Here's how the part is built. I have some questions about the finished solid (model axes, mm). Face numbers are marked on the shaded views. A direction names the side the tool comes from. Round coordinates to 2 decimals unless told otherwise and drop trailing zeros. Loops run counter-clockwise (first coordinate to the right, second up) from the corner with the lowest first, then second, coordinate; pieces in that order, holes last. Notation, with made-up numbers: M -36,-23 L 11,-23 A26 cw 11,-4 Z; hole C 19,39.25 d3. An arc over 180 degrees is marked long. Answer as a JSON object with one key per item and string values.
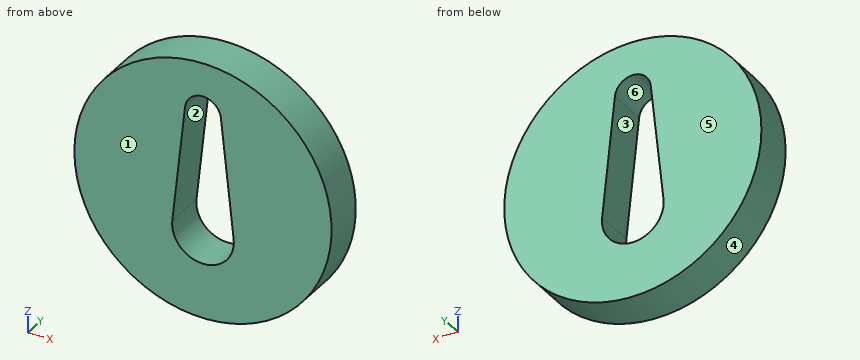
Autodesk Inventor part; units mm, degrees
ref_plane "YZ Plane" through (0, 0, 0) normal (1, 0, 0) x (0, 1, 0)
ref_plane "XZ Plane" through (0, 0, 0) normal (0, 1, 0) x (-1, 0, 0)
ref_plane "XY Plane" through (0, 0, 0) normal (0, 0, 1) x (1, 0, 0)
sketch "Sketch1" plane through (0, 0, 0) normal (0, 1, 0) x (-1, 0, 0)
  circle A0 centre (0, 0) radius 20 construction
  circle A1 centre (0, 5) radius 15
  circle A2 centre (0, 0) radius 3.5
  circle A3 centre (0, 14) radius 2
  line L0 (-1.9885, 14.2143) -> (-3.4799, 0.375)
  line L1 (1.9885, 14.2143) -> (3.4799, 0.375)
  dimension "d0" = 40
  dimension "d1" = 30
  dimension "d2" = 7
  dimension "d3" = 4
  dimension "d4" = 19.5
extrude "Extrusion1" add sketch "Sketch1" along normal blind 4.8
sketch "Sketch2" plane through (0, 4.8, 5) normal (0, 1, 0) x (1, 0, 0)
  arc A0 (-1.9885, -9.2143) -> (1.9885, -9.2143) centre (0, -9) ccw
  line L0 (1.9885, -9.2143) -> (3.4799, 4.625)
  arc A1 (3.4799, 4.625) -> (-3.4799, 4.625) centre (0, 5) ccw
  line L1 (-3.4799, 4.625) -> (-1.9885, -9.2143)
  circle A2 centre (0, 0) radius 15
  arc A3 (-2.0879, -9.225) -> (2.0879, -9.225) centre (0, -9) ccw
  line L2 (2.0879, -9.225) -> (3.5793, 4.6143)
  arc A4 (3.5793, 4.6143) -> (-3.5793, 4.6143) centre (0, 5) ccw
  line L3 (-3.5793, 4.6143) -> (-2.0879, -9.225)
  dimension "d7" = 0.1
extrude "Extrusion2" cut sketch "Sketch2" against normal through all contours L3 A4 L2 A3
properties part number "Ventil Scheibe_3DPrint"
Item 1: I want a section at B-B on x = 0. List the corners of the cut face in (y, z) for me, plus the area to 3 significant figures.
Solution:
{"outline": "M 0,-10 L 4.8,-10 L 4.8,-3.6 L 0,-3.6 Z; M 0,16.1 L 4.8,16.1 L 4.8,20 L 0,20 Z", "area": "49.4 mm2"}
Item 2: We'd pull the mould along Z, two halves only. Please class the marked faces 1, 2, 3 and 4: +Z half, -Z half, draft (parallel to the pull), parting line (faces both ways), or undercut.
Solution:
{"face 1": "draft", "face 2": "undercut", "face 3": "undercut", "face 4": "parting line"}
Item 3: If I drill on L1, parallel to X at y = 1.5, z = 13.5; L2, parallel to X at y = 3.25, z = 0; L3, parallel to Z at x = 10, y = 1.3, over which ranges is the centre line in solid material (lowest first)? Write a range as from..to.
Solution:
{"L1": "x = -12.36..-2.17, 2.17..12.36", "L2": "x = -14.14..-3.6, 3.6..14.14", "L3": "z = -6.18..16.18"}
Item 4: For P1, Ø2, axis at x = 6, y = 3.5, coming from the -Z side, with a flat end and sliding along its axis, tell me the tip position at first contact or that it passes through.
Solution:
{"P1": "stops at z = -9.14"}
Item 5: I want a section at D-D on z = -7. List the corners of the cut face in (x, y) for me.
Solution:
{"outline": "M -9,0 L 9,0 L 9,4.8 L -9,4.8 Z"}
Item 6: I want a section at C-C on y = 4.15. List the corners of the cut face in (x, z) for me (3 decimals).
Solution:
{"outline": "C 0,5 d30; hole M -3.579,0.386 A3.6 ccw long 3.579,0.386 L 2.088,14.225 A2.1 ccw -2.088,14.225 Z"}
Item 7: I want a section at A-A on z = 12.75. List the corners of the cut face in (x, y) for me.
Solution:
{"outline": "M -12.84,0 L -2.25,0 L -2.25,4.8 L -12.84,4.8 Z; M 2.25,0 L 12.84,0 L 12.84,4.8 L 2.25,4.8 Z"}
Item 8: For the marked faces 5 and 6, which set-ups out of +Z, -Z, +X, -X, +Y, -Y let a thin tool reach every point of the face, with its end or its side?
Solution:
{"face 5": "+Z, -Z, +X, -X, +Y", "face 6": "+Y, -Y"}
